Build history of the part. All positions in model axes, mm. A direction names the side the tool comes from. Round coordinates to 2 decimals unless told otherwise and drop trailing zeros. Loops run counter-clockwise (first coordinate to the right, second up) from the corner with the lowest first, then second, coordinate; pieces in that order, holes last. Notation, with made-up numbers: (-9.75, -35.5) -> (4.25, -35.5) arc R18 cw to (4.25, -9.5) -> close; hole circle Ø8 at (-26, -29). An arc over 180 degrees is marked (long way). Put each result on its own line as item: value. Start each with the question number.
Solid Edge part; units mm, degrees
sketch "Sketch1" plane through (0, 0, 0) normal (0, 0, 1) x (1, 0, 0)
  line L0 (23, -69.5) -> (-23, -69.5)
  line L1 (-23, -69.5) -> (-23, 69.5)
  line L2 (-23, 69.5) -> (23, 69.5)
  line L3 (23, 69.5) -> (23, -69.5)
  dimension "D1" = 23
  dimension "D2" = 23
extrude "Protrusion1" add sketch "Sketch1" along normal blind 49
fillet "Verrundung_2" radius 2 12 edges at (-23, 0, 0) (0, -69.5, 0) (23, 0, 0) (0, 69.5, 0) (23, 69.5, 24.5) (-23, 69.5, 24.5) (0, 69.5, 49) (23, 0, 49) (23, -69.5, 24.5) (0, -69.5, 49) (-23, -69.5, 24.5) (-23, 0, 49)
sketch "Sketch2" plane through (0, 0, 49) normal (0, 0, 1) x (1, 0, 0)
  circle A0 centre (-17.5, 64) radius 2.5
extrude "Extrusionsausschnitt_1" cut sketch "Sketch2" against normal blind 10
mirror "Mirror1" about plane through (0, 0, 0) normal (1, 0, 0) of "Extrusionsausschnitt_1"
sketch "Sketch3" plane through (0, 0, 49) normal (0, 0, 1) x (-1, 0, 0)
  line L0 (-5, -61.5) -> (5, -61.5)
  line L1 (-5, -66.5) -> (5, -66.5)
  arc A0 (-5, -66.5) -> (-5, -61.5) centre (-5, -64) cw
  arc A1 (5, -61.5) -> (5, -66.5) centre (5, -64) cw
  dimension "D1" = 5
extrude "Extrusionsausschnitt_3" cut sketch "Sketch3" against normal blind 10
fillet "Verrundung_3" radius 0.5 6 edges at (-20, 64, 49) (-7.5, 64, 49) (0, 66.5, 49) (7.5, 64, 49) (0, 61.5, 49) (20, 64, 49)
Item 1: Pull direction X, two halves, no side cores. Call faces 3 (the face through (23, 1, 24)), 4 (the face through (-7.5, 64.1, 43.8)), 5 (the face through (0, 1, 0)), 6 (the face through (-18, 64, 39)): +X half, -X half, draft (parallel to the pull), parting line (faces both ways), or undercut.
Item 2: Wall check: line 1 (Y direction, x = 17.5, z = 43.25); line 2 (Y direction, x = 17, z = 39.5). Give the ranges that are in metal, low to high. Write a range as from..to.
Item 3: Drop flat-ended pins along their axis: pin 1 (4.5 mm diameter, centred on x = 17.5, y = 64, fed in from +Z); pin 2 (2.5 mm diameter, centred on x = -16.5, y = 65, fed in from +Z). Give the stop position or say it passes through.
Item 4: 3-axis set-ups, long thin cutter, end or side, ignore diameter. For faces 1 (the face through (0, 69.5, 24)), 2 (the face through (-20, 64, 44)): which of +Z, -Z, +X, -X, +Y, -Y reach the whole face in a straight line?
Item 5: Cut at A-A on y = 64. Write the cut outline in (x, z), then the cut area to 3 significant figures.
Ans:
1. face 3: +X half
1. face 4: undercut
1. face 5: draft
1. face 6: undercut
2. line 1: y = -69.5..61.5, 66.5..69.5
2. line 2: y = -69.5..61.55, 66.45..69.5
3. pin 1: stops at z = 39
3. pin 2: stops at z = 48.87
4. face 1: +Z, -Z, +X, -X, +Y
4. face 2: +Z
5. outline: (-23, 2) arc R2 ccw to (-21, 0) -> (21, 0) arc R2 ccw to (23, 2) -> (23, 47) arc R2 ccw to (21, 49) -> (20.5, 49) arc R0.5 ccw to (20, 48.5) -> (20, 39) -> (15, 39) -> (15, 48.5) arc R0.5 ccw to (14.5, 49) -> (8, 49) arc R0.5 ccw to (7.5, 48.5) -> (7.5, 39) -> (-7.5, 39) -> (-7.5, 48.5) arc R0.5 ccw to (-8, 49) -> (-14.5, 49) arc R0.5 ccw to (-15, 48.5) -> (-15, 39) -> (-20, 39) -> (-20, 48.5) arc R0.5 ccw to (-20.5, 49) -> (-21, 49) arc R2 ccw to (-23, 47) -> close
5. area: 2,000 mm2
